Geometry check sheet. Reference: drawing and pictorial views, mm from the part's lowest x, y, z. Give positions to 0.01 mm unless a question says otherwise; leave off trailing zeros. Order: outer loops, then holes, each group sorted by start corner. A loop starts at its lowest first (then second) coordinate and runs counter-clockwise, first axis right, second up.
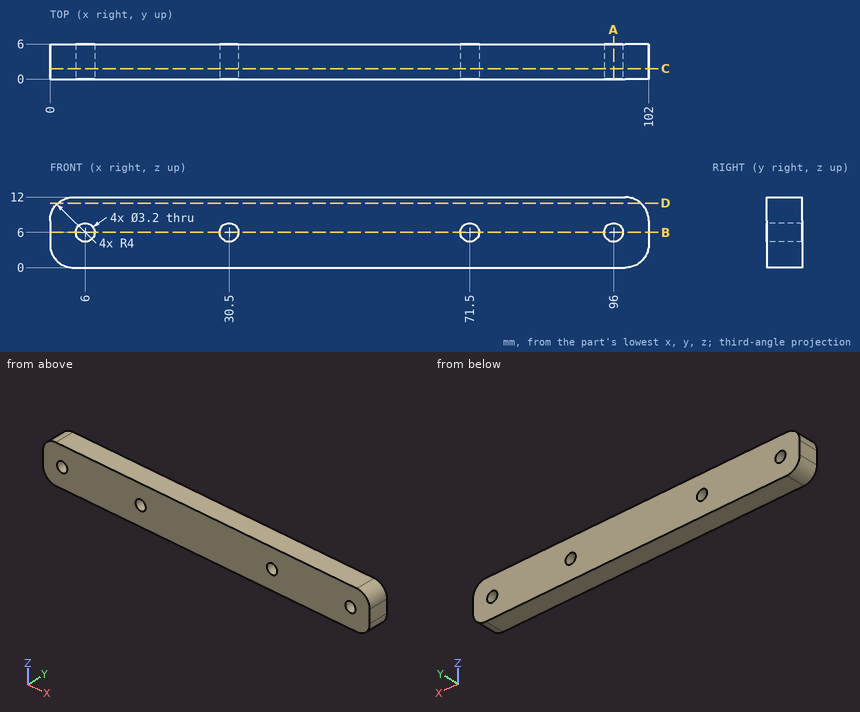
(1) Cross-section at B-B on z = 6. Enter the section's corners in (x, y), then the cut area to 3 significant figures.
Response values:
outline: (0, 0) - (4.4, 0) - (4.4, 6) - (0, 6) - close; (7.6, 0) - (28.9, 0) - (28.9, 6) - (7.6, 6) - close; (32.1, 0) - (69.9, 0) - (69.9, 6) - (32.1, 6) - close; (73.1, 0) - (94.4, 0) - (94.4, 6) - (73.1, 6) - close; (97.6, 0) - (102, 0) - (102, 6) - (97.6, 6) - close
area: 535 mm2
(2) Cross-section at A-A on x = 96. Enter the section's corners in (y, z).
Response values:
outline: (0, 0) - (6, 0) - (6, 4.4) - (0, 4.4) - close; (0, 7.6) - (6, 7.6) - (6, 12) - (0, 12) - close
(3) Material ranges on L1, parallel to X at y = 2.95, z = 6; L2, parallel to X at y = 3, z = 7.25; L3, parallel to Z at x = 71.5, y = 4.4, recorded low to high.
Response values:
L1: x = 0 to 4.4, 7.6 to 28.9, 32.1 to 69.9, 73.1 to 94.4, 97.6 to 102
L2: x = 0 to 5, 7 to 29.5, 31.5 to 70.5, 72.5 to 95, 97 to 102
L3: z = 0 to 4.4, 7.6 to 12
(4) Cross-section at C-C on y = 1.8. Enter the section's corners in (x, z), then the cut area to 3 significant figures.
Response values:
outline: (0, 4) arc R4 ccw to (4, 0) - (98, 0) arc R4 ccw to (102, 4) - (102, 8) arc R4 ccw to (98, 12) - (4, 12) arc R4 ccw to (0, 8) - close; hole circle Ø3.2 at (6, 6); hole circle Ø3.2 at (30.5, 6); hole circle Ø3.2 at (71.5, 6); hole circle Ø3.2 at (96, 6)
area: 1,180 mm2
(5) Cross-section at D-D on z = 11. Enter the section's corners in (x, y).
Response values:
outline: (1.35, 0) - (100.65, 0) - (100.65, 6) - (1.35, 6) - close
(6) Gauge pin test, flat end, axial feed: pin 1 Ø1 at (y, z) = (3, 1.5) entering from +X. Record the tip position at first contact, or that the pin passes through.
Response values:
pin 1: stops at x = 101.46
